The figure shows three views and two pictorial views of one solid part (mm, origin at its lowest corner). Answer the questions. Coordinates: 2 decimals unless noted, no trailing zeros. Write each loop counter-clockwise with the first axis right and the second up, starting at its lowest first coordinate (ties: lowest second). Pieces come first, ordered by that corner, then holes.
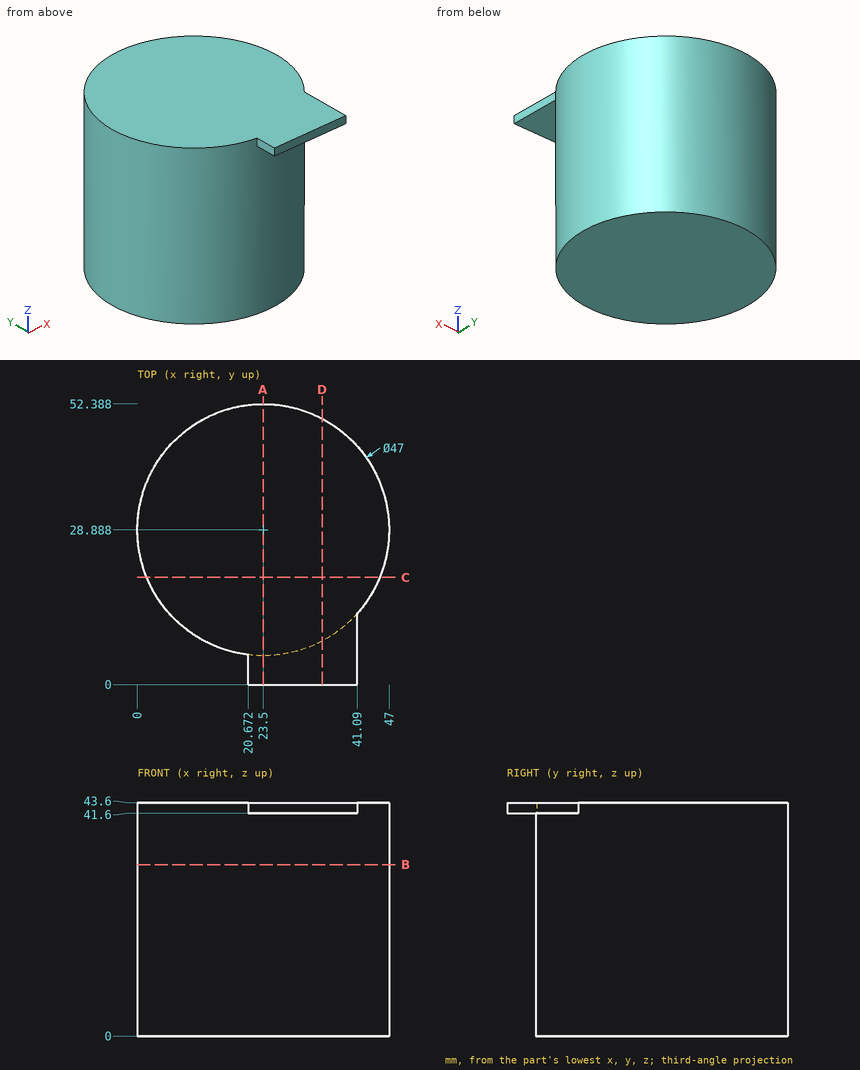
1. Section D-D on x = 34.5 is taken. Give the vertices of the cut face in (y, z) (1 decimal), then the cut area to 3 significant figures.
Results found:
outline: (0, 41.6) - (8.1, 41.6) - (8.1, 0) - (49.7, 0) - (49.7, 43.6) - (0, 43.6) - close
area: 1,830 mm2
2. Flat-ended cylindrical pins translate along their axes: P1, Ø8, axis at x = 32, z = 11.5, coming from the +Y side; P2, Ø1.6, axis at y = 8.5, z = 42.5, coming from the +X side; P3, Ø2, axis at y = 19, z = 30.5, coming from the -X side (1 decimal). Find the tip coordinate at first contact, or state that the pin passes through.
Results found:
P1: stops at y = 51.95
P2: stops at x = 41.09
P3: stops at x = 1.7
3. Find the intervals of material crossed by L1, parallel to Y at x = 35, z = 11 (1 decimal); L2, parallel to X at y = 32.5, z = 9; L3, parallel to X at y = 26.5, z = 13, in increasing order.
Results found:
L1: y = 8.4 to 49.4
L2: x = 0.28 to 46.72
L3: x = 0.12 to 46.88
4. Section C-C on y = 20 is taken. Give the vertices of the cut face in (x, z) (1 decimal).
Results found:
outline: (1.7, 0) - (45.3, 0) - (45.3, 43.6) - (1.7, 43.6) - close
5. Section A-A on x = 23.5 is taken. Give the vertices of the cut face in (y, z).
Results found:
outline: (0, 41.6) - (5.39, 41.6) - (5.39, 0) - (52.39, 0) - (52.39, 43.6) - (0, 43.6) - close
6. Section B-B on z = 32 is taken. Give the vertices of the cut face in (x, y), then the cut area to 4 significant figures.
Results found:
outline: circle Ø47 at (23.5, 28.89)
area: 1,735 mm2
